Here's how the part is built. I have some questions about the finished solid (model axes, mm). Face numbers are marked on the shaded views. A direction names the side the tool comes from. Give positions to 0.01 mm unless a question says otherwise; leave off trailing zeros. Order: outer loops, then holes, each group sorted by start corner. A loop starts at its lowest first (then second) coordinate and runs counter-clockwise, first axis right, second up. Notation, with made-up numbers: M 40,-33 L 78,-33 A23 cw 78,-13 Z; hole C 86,18 d5. An arc over 180 degrees is marked long. Use one line per item in the form item = value.
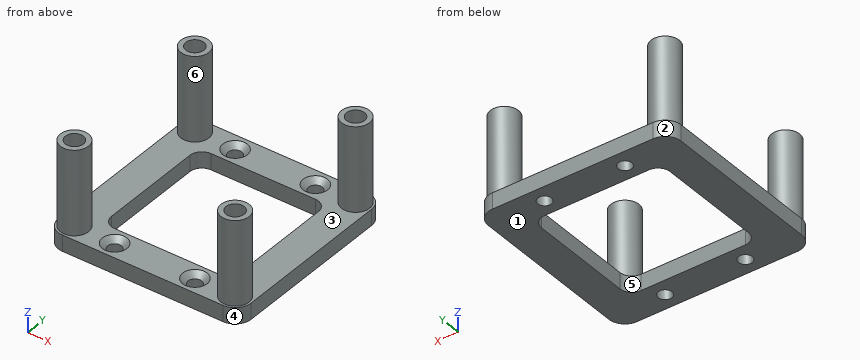
from build123d import *

# Parameters (mm, degrees)
SKETCH005_R                        = 3.5
PAD003_DEPTH                       = 25
SKETCH007_W                        = 48
SKETCH007_H                        = 48
SKETCH007_W_2                      = 32
SKETCH007_H_2                      = 32
PAD004_DEPTH                       = 4
SKETCH006_R                        = 2.25
POCKET001_DEPTH                    = 7
SKETCH005_LINEARPATTERN002_2_R     = 3.5
PAD003_LINEARPATTERN002_2_DEPTH    = 25
SKETCH006_LINEARPATTERN002_2_R     = 2.25
POCKET001_LINEARPATTERN002_2_DEPTH = 7
LINEARPATTERN003_COUNT             = 2
LINEARPATTERN003_PITCH             = 40
HOLE001_D                          = 3.4
HOLE001_DEPTH                      = 25
HOLE001_CSINK_D                    = 6.1
HOLE001_CSINK_ANGLE                = 90
FILLET002_R                        = 4
FILLET003_R                        = 3


with BuildPart() as part:
    # Sketch005 → Pad003 (new body)
    with BuildSketch(Plane.XY):
        Circle(SKETCH005_R)
    pad003 = extrude(amount=PAD003_DEPTH)

    # Sketch007 → Pad004 (join)
    with BuildSketch(Plane.XY):
        with Locations((20, 20)):
            Rectangle(SKETCH007_W, SKETCH007_H)
        with Locations((20, 20)):
            Rectangle(SKETCH007_W_2, SKETCH007_H_2, mode=Mode.SUBTRACT)
    extrude(amount=PAD004_DEPTH)

    # Sketch006 → Pocket001 (cut)
    with BuildSketch(Plane.XY.offset(25)):
        Circle(SKETCH006_R)
    pocket001 = extrude(amount=-POCKET001_DEPTH, mode=Mode.SUBTRACT)

    # Sketch005 LinearPattern002 2 → Pad003 LinearPattern002 2 (add)
    with BuildSketch(Plane(origin=(40, 0, 0), x_dir=(1, 0, 0), z_dir=(0, 0, 1))):
        Circle(SKETCH005_LINEARPATTERN002_2_R)
    pad003_linearpattern002_2 = extrude(amount=PAD003_LINEARPATTERN002_2_DEPTH)

    # Sketch006 LinearPattern002 2 → Pocket001 LinearPattern002 2 (cut)
    with BuildSketch(Plane(origin=(40, 0, 25), x_dir=(1, 0, 0), z_dir=(0, 0, 1))):
        Circle(SKETCH006_LINEARPATTERN002_2_R)
    pocket001_linearpattern002_2 = extrude(amount=-POCKET001_LINEARPATTERN002_2_DEPTH, mode=Mode.SUBTRACT)

    # LinearPattern003: Pad003, Pocket001, Pad003 LinearPattern002 2, Pocket001 LinearPattern002 2 ×2
    with Locations(*[(0, i * LINEARPATTERN003_PITCH, 0) for i in range(1, LINEARPATTERN003_COUNT)]):
        add(pad003)
        add(pocket001, mode=Mode.SUBTRACT)
        add(pad003_linearpattern002_2)
        add(pocket001_linearpattern002_2, mode=Mode.SUBTRACT)

    # Hole001
    with Locations(Plane.XY.offset(4)):
        with Locations((10, 40), (30, 40), (30, 0), (10, 0)):
            CounterSinkHole(HOLE001_D / 2, HOLE001_CSINK_D / 2, depth=HOLE001_DEPTH, counter_sink_angle=HOLE001_CSINK_ANGLE)

    # Fillet002
    fillet002_edges = [part.edges().sort_by_distance(p)[0] for p in [
        (-4, -4, 2),
        (44, -4, 2),
        (-4, 44, 2),
        (44, 44, 2),
    ]]
    fillet(fillet002_edges, radius=FILLET002_R)

    # Fillet003
    fillet003_edges = [part.edges().sort_by_distance(p)[0] for p in [
        (4, 36, 2),
        (36, 36, 2),
        (36, 4, 2),
        (4, 4, 2),
    ]]
    fillet(fillet003_edges, radius=FILLET003_R)


solid = part.part
Q1. I want a section at C-C on x = 30. Write out the boundary of the cut face in (y, z), then the cut area to 3 significant figures.
Found:
outline = M -4,0 L -1.7,0 L -1.7,2.65 L -3.05,4 L -4,4 Z; M 1.7,0 L 4,0 L 4,4 L 3.05,4 L 1.7,2.65 Z; M 36,0 L 38.3,0 L 38.3,2.65 L 36.95,4 L 36,4 Z; M 41.7,0 L 44,0 L 44,4 L 43.05,4 L 41.7,2.65 Z
area = 33.2 mm²
Q2. On a 3-axis mill with a long thin cutter (end or side, diameter ignored), from which of +Z, -Z, +X, -X, +Y, -Y can I reach the whole of each face in a straight line? I mean the marked faces 5 and 6. Say none if no direction works.
Found:
face_5 = +Z, -Z
face_6 = +Z
Q3. Thinking about a two-plate mould opening in X: for the marked faces 1, 2, 3 and 4, which applies, +X half, -X half, draft (parallel to the pull), parting line (faces both ways), or undercut?
Found:
face_1 = draft
face_2 = -X half
face_3 = undercut
face_4 = +X half
Q4. I need wall thicknesses on L1, parallel to Y at x = 0, z = 21; L2, parallel to X at y = 0, z = 1.2; L3, parallel to X at y = 23, z = 3.5. Which ranges of each line are inside material? Lowest first, please.
Found:
L1 = -3.5 to -2.25, 2.25 to 3.5, 36.5 to 37.75, 42.25 to 43.5
L2 = -4 to 8.3, 11.7 to 28.3, 31.7 to 44
L3 = -4 to 4, 36 to 44
Q5. I want a section at B-B on y = 24.5. Write out the boundary of the cut face in (x, z).
Found:
outline = M -4,0 L 4,0 L 4,4 L -4,4 Z; M 36,0 L 44,0 L 44,4 L 36,4 Z
Q6. I want a section at A-A on z = 20.5. Write out the boundary of the cut face in (x, y).
Found:
outline = C 0,0 d7; C 0,40 d7; C 40,0 d7; C 40,40 d7; hole C 0,0 d4.5; hole C 0,40 d4.5; hole C 40,0 d4.5; hole C 40,40 d4.5
Q7. I'm going to push flat-ended pins straight in: pin 1 Ø1.3 at (x, y) = (40, 39) entering from +Z; pin 2 Ø7 at (x, y) = (0, 0) entering from +Z; pin 3 Ø8 at (y, z) = (34.5, 18) entering from +X; pin 4 Ø5.5 at (x, y) = (30, 40) entering from +Z. Where does each tip first touch, or does it pass through?
Found:
pin_1 = 18
pin_2 = 25
pin_3 = 43.16
pin_4 = 3.7
